```python
from build123d import *

# Parameters (mm, degrees)
SKETCH1_W                                  = 41
SKETCH1_H                                  = 51
BOSS_EXTRUDE1_DEPTH                        = 3
SKETCH2_W                                  = 37
SKETCH2_H                                  = 47
CUT_EXTRUDE1_DEPTH                         = 2
SKETCH4_R                                  = 1.75
BOSS_EXTRUDE2_DEPTH                        = 3
MIRROR1_AT_THE_SECOND_PLANE_COPY_1_SKETC_R = 1.75
MIRROR1_AT_THE_SECOND_PLANE_COPY_1_DEPTH   = 3


with BuildPart() as part:
    # Sketch1 → Boss-Extrude1 (new body)
    with BuildSketch(Plane.XY):
        Rectangle(SKETCH1_W, SKETCH1_H)
    extrude(amount=BOSS_EXTRUDE1_DEPTH)

    # Sketch2 → Cut-Extrude1 (cut)
    with BuildSketch(Plane.XY.offset(3)):
        Rectangle(SKETCH2_W, SKETCH2_H)
    extrude(amount=-CUT_EXTRUDE1_DEPTH, mode=Mode.SUBTRACT)

    # Sketch4 → Boss-Extrude2 (add)
    with BuildSketch(Plane.XY):
        with BuildLine():
            Line((25.5, 25.5), (20.5, 25.5))
            Line((20.5, 25.5), (20.5, 12.5))
            Line((20.5, 12.5), (27.967226295, 18.351540947))
            ThreePointArc((27.967226295, 18.351540947), (29.281126566, 22.805021798), (25.5, 25.5))
        make_face()
        with Locations((25.5, 21.5)):
            Circle(SKETCH4_R, mode=Mode.SUBTRACT)
    boss_extrude2 = extrude(amount=BOSS_EXTRUDE2_DEPTH)

    # Mirror1: Boss-Extrude2 across plane
    add(boss_extrude2.mirror(Plane(origin=(0, 0, 0), x_dir=(0, 0, 1), z_dir=(1, 0, 0))))

    # Mirror1 at the second plane: Boss-Extrude2 across plane
    add(boss_extrude2.mirror(Plane.ZX))

    # Mirror1 at the second plane copy 1 sketc → Mirror1 at the second plane copy 1 (add)
    with BuildSketch(Plane(origin=(0, 0, 0), x_dir=(-1, 0, 0), z_dir=(0, 0, 1))):
        with BuildLine():
            Line((25.5, 25.5), (20.5, 25.5))
            Line((20.5, 25.5), (20.5, 12.5))
            Line((20.5, 12.5), (27.967226295, 18.351540947))
            ThreePointArc((27.967226295, 18.351540947), (29.281126566, 22.805021798), (25.5, 25.5))
        make_face()
        with Locations((25.5, 21.5)):
            Circle(MIRROR1_AT_THE_SECOND_PLANE_COPY_1_SKETC_R, mode=Mode.SUBTRACT)
    extrude(amount=MIRROR1_AT_THE_SECOND_PLANE_COPY_1_DEPTH)


solid = part.part
```
Design review of the part built by this model. Coordinates are the model's own, in mm. A direction names the side the tool comes from. Coordinates: 2 decimals unless noted, no trailing zeros. Order: outer loops, then holes, each group sorted by start corner. A loop starts at its lowest first (then second) coordinate and runs counter-clockwise, first axis right, second up. Notation, with made-up numbers: (15.5, 0.25) - (19.5, 0.25) arc R8 cw to (19.5, 5.25) - close; hole circle Ø1 at (-27, 57.5). An arc over 180 degrees is marked (long way). Answer in a Markdown table with one row per item.
(1) Wall thickness on line 1 along X through (y, z) = (-21.5, 0.8); line 2 along X through (y, z) = (3, 2.15); line 3 along Y through (x, z) = (0.5, 1.1): over which ranges is each line inside the solid? List them lowest first. Write a range as from..to.
Checked values:
| item | result |
|---|---|
| line 1 | -29.5..-27.25, -23.75..23.75, 27.25..29.5 |
| line 2 | -20.5..-18.5, 18.5..20.5 |
| line 3 | -25.5..-23.5, 23.5..25.5 |
(2) Consider section D-D on y = 5. State the section outline as (x, z) points.
Checked values:
| item | result |
|---|---|
| outline | (-20.5, 0) - (20.5, 0) - (20.5, 3) - (18.5, 3) - (18.5, 1) - (-18.5, 1) - (-18.5, 3) - (-20.5, 3) - close |
(3) Consider section A-A on y = -21.5. State the section outline as (x, z) points, plus the area to 3 significant figures.
Checked values:
| item | result |
|---|---|
| outline | (-29.5, 0) - (-27.25, 0) - (-27.25, 3) - (-29.5, 3) - close; (-23.75, 0) - (23.75, 0) - (23.75, 3) - (18.5, 3) - (18.5, 1) - (-18.5, 1) - (-18.5, 3) - (-23.75, 3) - close; (27.25, 0) - (29.5, 0) - (29.5, 3) - (27.25, 3) - close |
| area | 82.0 mm^2 |
(4) Consider section C-C on x = -0.5. State the section outline as (y, z) points, plus the area to 3 significant figures.
Checked values:
| item | result |
|---|---|
| outline | (-25.5, 0) - (25.5, 0) - (25.5, 3) - (23.5, 3) - (23.5, 1) - (-23.5, 1) - (-23.5, 3) - (-25.5, 3) - close |
| area | 59.0 mm^2 |
(5) Clearance check with flat-ended pins moving along their axes: pin 1 (1 mm diameter, centred on y = 14.5, z = 1.5, fed in from +X); pin 2 (3 mm diameter, centred on x = -25.5, y = -21.5, fed in from -Z); pin 3 (8 mm diameter, centred on x = -20, y = -6.5, fed in from -Z); pin 4 (1.6 mm diameter, centred on y = -7.5, z = 1.5, fed in from +X). State where each tip first meets the part, or that it passes through.
Checked values:
| item | result |
|---|---|
| pin 1 | x = 23.69 |
| pin 2 | through |
| pin 3 | z = 0 |
| pin 4 | x = 20.5 |
(6) For faces 4 (the flat face through (-20.5, 0, 1)), 5 (the flat face through (0, 23.5, 2)), 6 (the flat face through (0, 25.5, 1)), 7 (the flat face through (24.2, 15.4, 1.5)), list the 3-axis set-ups (+Z, -Z, +X, -X, +Y, -Y) from which the entire face can be reached by the end or side of a thin tool; tool diameter is ignored.
Checked values:
| item | result |
|---|---|
| face 4 | +Z, -Z, -X |
| face 5 | +Z |
| face 6 | +Z, -Z, +X, -X, +Y |
| face 7 | +Z, -Z, +X |
(7) Consider section B-B on z = 1.85. State the section outline as (x, y) points, plus the area to 3 significant figures.
Checked values:
| item | result |
|---|---|
| outline | (-27.97, -18.35) arc R4 ccw to (-25.5, -25.5) - (25.5, -25.5) arc R4 ccw to (27.97, -18.35) - (20.5, -12.5) - (20.5, 12.5) - (27.97, 18.35) arc R4 ccw to (25.5, 25.5) - (-25.5, 25.5) arc R4 ccw to (-27.97, 18.35) - (-20.5, 12.5) - (-20.5, -12.5) - close; hole circle Ø3.5 at (-25.5, -21.5); hole circle Ø3.5 at (-25.5, 21.5); hole (-18.5, -23.5) - (18.5, -23.5) - (18.5, 23.5) - (-18.5, 23.5) - close; hole circle Ø3.5 at (25.5, -21.5); hole circle Ø3.5 at (25.5, 21.5) |
| area | 639 mm^2 |
(8) The part is to be moulded in two halves that separate along X. For faces 1 (the flat face through (24.2, -15.4, 1.5)), 2 (the cylindrical face through (-29.303, -22.739, 1.479)), 3 (the flat face through (18.5, 0, 2)), say which applies: released by +X, released by -X, zero draft, split by the parting line, or undercut.
Checked values:
| item | result |
|---|---|
| face 1 | released by +X |
| face 2 | released by -X |
| face 3 | undercut |
